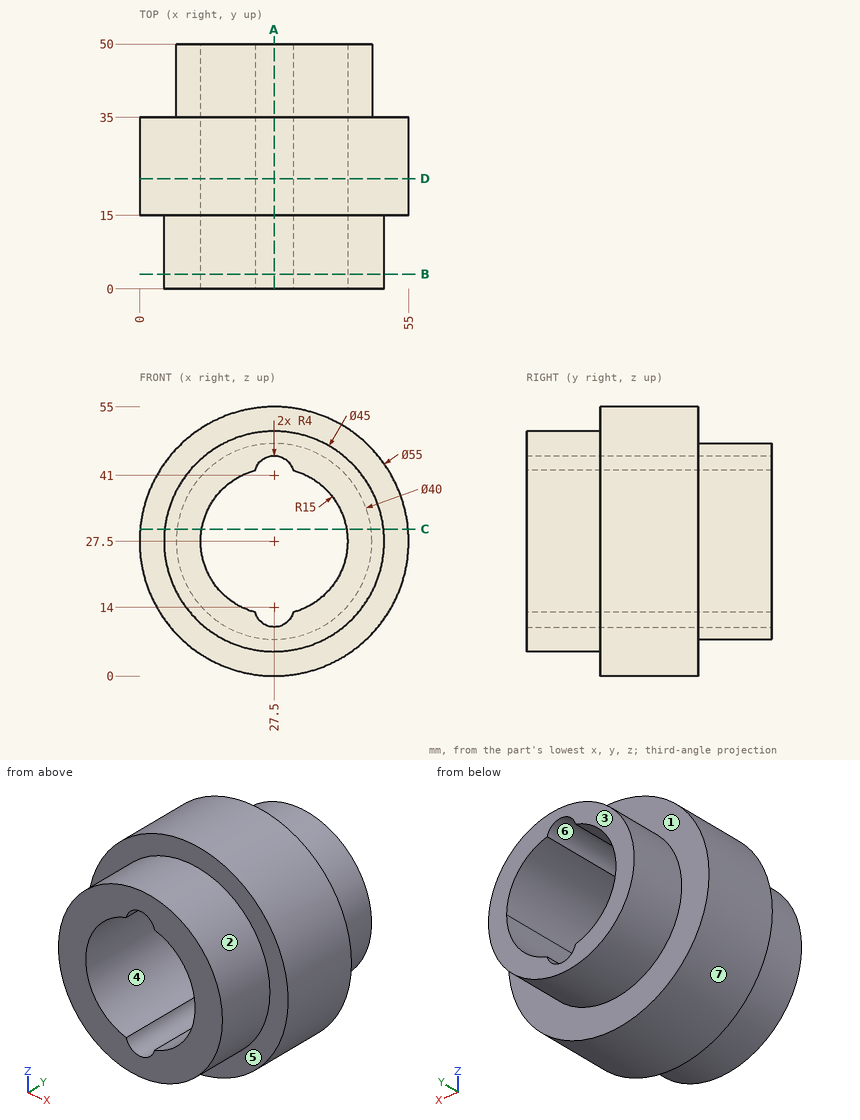
Can you work these out from the drawing? Everything is in mm from the part's minimum corner. A direction names the side the tool comes from. Round coordinates to 2 decimals unless told otherwise and drop trailing zeros. Write each loop counter-clockwise with the first axis right and the second up, starting at its lowest first coordinate (ties: lowest second). Pieces come first, ordered by that corner, then holes. Notation, with made-up numbers: (-2, 19.5) - (23, 19.5) arc R22 ccw to (23, 47.5) - close; hole circle Ø5 at (9, 68.25). An arc over 180 degrees is marked (long way). Use a Markdown table: item, result.
Q1. I want a section at C-C (z = 30). List the corners of the cut face in (x, y) for me, plus the area to 3 significant figures.
Output values:
| item | result |
|---|---|
| outline | (0.11, 15) - (5.14, 15) - (5.14, 0) - (12.71, 0) - (12.71, 50) - (7.66, 50) - (7.66, 35) - (0.11, 35) - close; (42.29, 0) - (49.86, 0) - (49.86, 15) - (54.89, 15) - (54.89, 35) - (47.34, 35) - (47.34, 50) - (42.29, 50) - close |
| area | 883 mm2 |
Q2. I want a section at D-D (y = 22.5). List the corners of the cut face in (x, z) for me.
Output values:
| item | result |
|---|---|
| outline | circle Ø55 at (27.5, 27.5); hole (23.62, 13.01) arc R4 ccw to (31.38, 13.01) arc R15 ccw to (42.5, 27.5) arc R15 ccw to (31.38, 41.99) arc R4 ccw to (23.62, 41.99) arc R15 ccw to start |
Q3. I want a section at B-B (y = 3). List the corners of the cut face in (x, z) for me, plus the area to 3 significant figures.
Output values:
| item | result |
|---|---|
| outline | circle Ø45 at (27.5, 27.5); hole (23.62, 13.01) arc R4 ccw to (31.38, 13.01) arc R15 ccw to (42.5, 27.5) arc R15 ccw to (31.38, 41.99) arc R4 ccw to (23.62, 41.99) arc R15 ccw to start |
| area | 854 mm2 |
Q4. For pin 1 (1 mm diameter, centred on y = 17.5, z = 44.5, fed in from -X); pin 2 (6 mm diameter, centred on x = 9.5, y = 35.5, fed in from -Z); pin 3 (6 mm diameter, centred on x = 20, y = 24, fed in from -Z), each with a flat end and sliding along its axis, tell me the tip position at first contact or that it passes through.
Output values:
| item | result |
|---|---|
| pin 1 | x = 5.5 |
| pin 2 | z = 4.48 |
| pin 3 | z = 0.37 |
Q5. I want a section at A-A (x = 27.5). List the corners of the cut face in (y, z) for me, plus the area to 3 significant figures.
Output values:
| item | result |
|---|---|
| outline | (0, 5) - (15, 5) - (15, 0) - (35, 0) - (35, 7.5) - (50, 7.5) - (50, 10) - (0, 10) - close; (0, 45) - (50, 45) - (50, 47.5) - (35, 47.5) - (35, 55) - (15, 55) - (15, 50) - (0, 50) - close |
| area | 625 mm2 |
Q6. Thinking about a two-plate mould opening in X: for the marked faces 5, 6 and 7, which applies, released by +X, released by -X, zero draft, split by the parting line, or undercut?
Output values:
| item | result |
|---|---|
| face 5 | zero draft |
| face 6 | undercut |
| face 7 | split by the parting line |
Q7. Please list where these lines run through material, in increasing order: L1, parallel to Z at x = 41, y = 47.5; L2, parallel to Z at x = 40, y = 34; L3, parallel to X at y = 40.5, z = 40.
Output values:
| item | result |
|---|---|
| L1 | 12.74 to 20.96, 34.04 to 42.26 |
| L2 | 3.01 to 19.21, 35.79 to 51.99 |
| L3 | 11.89 to 19.21, 35.79 to 43.11 |
Q8. For the marked faces 1, 2, 3 and 4, which set-ups out of +Z, -Z, +X, -X, +Y, -Y let a thin tool reach every point of the face, with its end or its side?
Output values:
| item | result |
|---|---|
| face 1 | +Y |
| face 2 | -Y |
| face 3 | +Z, -Z, +X, -X, +Y |
| face 4 | +Y, -Y |
